For this review, use the dimensioned drawing (mm, ordinates from the lowest corner) and the shaded views. Coordinates: 2 decimals unless noted, no trailing zeros. Order: outer loops, then holes, each group sorted by start corner. A loop starts at its lowest first (then second) coordinate and runs counter-clockwise, first axis right, second up. Notation, with made-up numbers: M 45.25,2 L 97.25,2 A11 cw 97.25,19 Z; hole C 47,83.5 d11. An arc over 180 degrees is marked long. Answer in a Markdown table with one row per item.
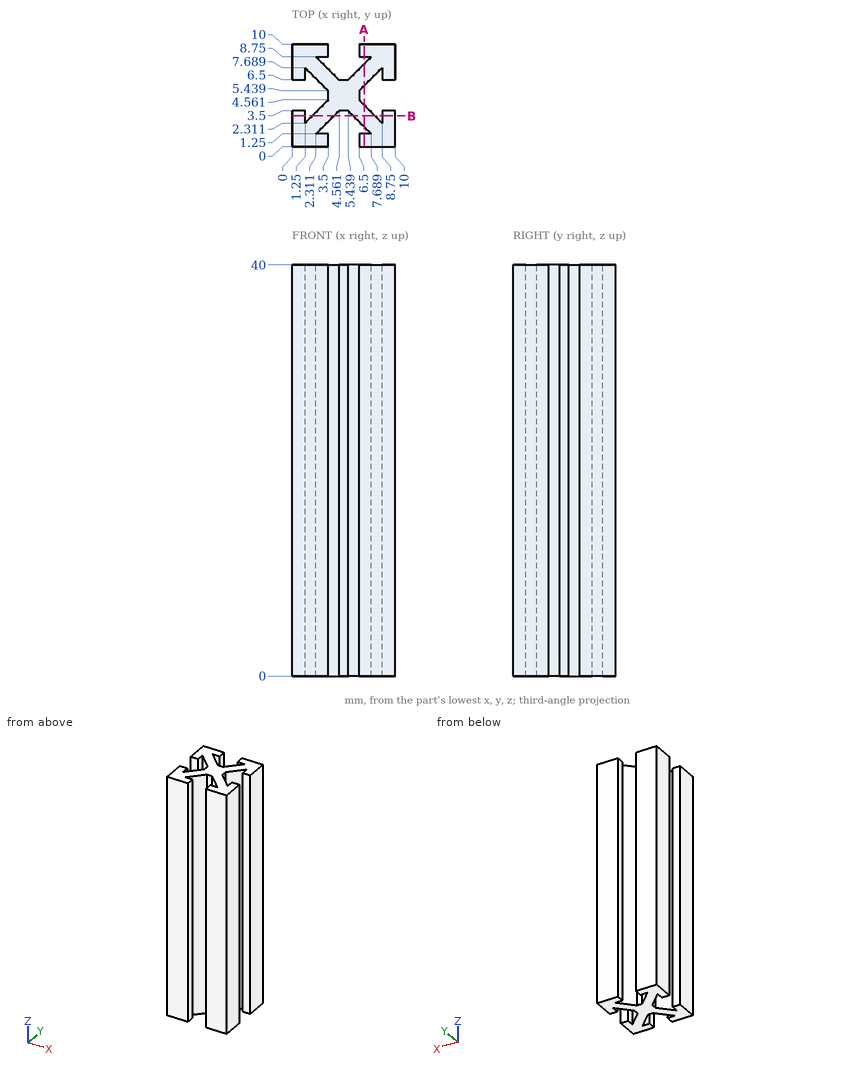
(1) Insertion check: P1, Ø1, axis at y = 5, z = 22, coming from the -X side. The pin has a flat end and moves straight along its axis. Give the tip position at first contact, or say it passes through.
Report:
| item | result |
|---|---|
| P1 | x = 3.44 |
(2) To check wall thickness, follow line 1 (X direction, y = 1, z = 19); line 2 (X direction, y = 2.5, z = 3). State the ranges of each line that lie inside material, in increasing order. Write a range as [from, to].
Report:
| item | result |
|---|---|
| line 1 | [0, 3.5], [6.5, 10] |
| line 2 | [0, 1.25], [1.44, 3.56], [6.44, 8.56], [8.75, 10] |
(3) Take a section at A-A (x = 7). Write out the cut boundary in (y, z).
Report:
| item | result |
|---|---|
| outline | M 0,0 L 1.25,0 L 1.25,40 L 0,40 Z; M 1.94,0 L 4.06,0 L 4.06,40 L 1.94,40 Z; M 5.94,0 L 8.06,0 L 8.06,40 L 5.94,40 Z; M 8.75,0 L 10,0 L 10,40 L 8.75,40 Z |
